Autodesk Inventor part; units mm, degrees
sketch "Skizze1" plane through (0, 0, 0) normal (0, 0, 1) x (1, 0, 0)
  line L0 (-9.4, 0) -> (56.4, 0)
  line L1 (0, -37.2) -> (0, 6.2)
  line L2 (0, 0) -> (47, 0)
  line L3 (47, 0) -> (47, -31)
  line L4 (47, -31) -> (0, -31)
  line L5 (0, -31) -> (0, 0)
  line L6 (5, -5) -> (42, -5)
  line L7 (42, -5) -> (42, -25)
  line L8 (42, -25) -> (39, -25)
  line L9 (39, -25) -> (39, -18)
  line L10 (39, -18) -> (8, -18)
  line L11 (8, -18) -> (8, -25)
  line L12 (8, -25) -> (5, -25)
  line L13 (5, -25) -> (5, -5)
  dimension "d0" = 47
  dimension "d1" = 31
  dimension "d2" = 5
  dimension "d3" = 5
  dimension "d4" = 5
  dimension "d5" = 6
  dimension "d6" = 6
  dimension "d7" = 3
  dimension "d8" = 3
  dimension "d9" = 13
extrude "Extrusion1" add sketch "Skizze1" along normal blind 50
fillet "Rundung1" radius 1 2 edges at (8, -18, 25) (39, -18, 25)
sketch "Skizze4" plane through (0, -31, 0) normal (-1, 0, 0) x (0, 0, 1)
  line L0 (50, 31) -> (50, 0)
  line L1 (0, 31) -> (50, 31)
  circle A0 centre (25, 17) radius 1.8
  dimension "d41" = 25
  dimension "d42" = 14
  dimension "d43" = 3.6
hole "Bohrung3" at (0, -14, 25) direction (1, 0, 0) diameter 6.15 end through all
sketch "Skizze5" plane through (0, 0, 0) normal (0, 1, 0) x (1, 0, 0)
  line L0 (0, 0) -> (47, 0)
  line L1 (0, 0) -> (10, 0)
  line L2 (10, 0) -> (10, -50)
  line L3 (10, -50) -> (0, -50)
  line L4 (0, -50) -> (0, 0)
  line L5 (47, 0) -> (47, -50)
  line L6 (47, 0) -> (37, 0)
  line L7 (37, 0) -> (37, -50)
  line L8 (37, -50) -> (47, -50)
  line L9 (47, -50) -> (47, 0)
  dimension "d51" = 10
  dimension "d52" = 50
  dimension "d53" = 10
  dimension "d54" = 50
extrude "Extrusion4" add sketch "Skizze5" along normal blind 10
sketch "Skizze6" plane through (47, -31, 50) normal (1, 0, 0) x (0, 0, -1)
  line L0 (0, 41) -> (50, 41)
  line L1 (50, 41) -> (50, 0)
  line L2 (0, 0) -> (0, 41)
  point P0 (50, 31)
  point P1 (12.5, 36)
  point P2 (25, 36)
  point P3 (37.5, 36)
  dimension "d57" = 5
  dimension "d58" = 5
  dimension "d59" = 5
  dimension "d60" = 12.5
  dimension "d61" = 12.5
  dimension "d62" = 12.5
hole "Bohrung4" at (47, 5, 37.5) at (47, 5, 25) at (47, 5, 12.5) direction (-1, 0, 0) diameter 6.15 end through all
properties part number "NASA Objektträgerhalter (Südkorea)"
Work out the finished part from the listing and answer in its coordinate system (mm). A direction names the side the tool comes from. Give positions to 0.01 mm unless a question says otherwise; leave off trailing zeros. Order: outer loops, then holes, each group sorted by start corner. A loop starts at its lowest first (then second) coordinate and runs counter-clockwise, first axis right, second up. Notation, with made-up numbers: (6.25, 43.5) - (24.25, 43.5) arc R15 cw to (24.25, 51.5) - close; hole circle Ø3 at (-11, -40). An arc over 180 degrees is marked (long way). Answer as CSV lines item,"result". Start each with the question number.
Q1. The part is cut by section C-C (z = 12.5). Write down the section's boundary in (x, y) (3 decimals), then the cut area to 3 significant figures.
Q2. Given pin 1 Ø8.5 at (x, z) = (24, 19) entering from +Y, flat-ended and moving along its own axis, determine where the tip first touches the part or whether it passes through.
Q3. The part is cut by section B-B (y = -8). Write down the section's boundary in (x, z).
Q4. The part is cut by section D-D (z = 4). Write down the section's boundary in (x, y), then the cut area to 3 significant figures.
Q5. The part is cut by section A-A (x = 41). Write down the section's boundary in (y, z) (3 decimals).
Q6. Find the intervals of material crossed by L1, parallel to Z at x = 6.5, y = 5 (3 decimals); L2, parallel to Y at x = 1.7, z = 25 (3 decimals); L3, parallel to X at y = -21, z = 7, in increasing order. Write a range as [from, to].
Q7. For faces 1 (the face through (7, -25, 25)), 2 (the face through (44.54, -14.14, 21.93)), 3 (the face through (37, 1.6, 24.7)), determine the directions among +Z, -Z, +X, -X, +Y, -Y from which every point of the face is accessible in a straight line to the end or side of a thin tool.
Q8. The mould has two halves that part along Y. Classify faces 4 (the face through (23, -19, 50)), 5 (the face through (24, -31, 25)), 6 (the face through (5, 10, 25)), 7 (the face through (24, -18, 25)): +Y half, -Y half, draft (parallel to the pull), parting line (faces both ways), or undercut.
Check result:
1,outline,"(0, -31) - (47, -31) - (47, 1.925) - (37, 1.925) - (37, 0) - (10, 0) - (10, 1.925) - (0, 1.925) - close; (0, 8.075) - (10, 8.075) - (10, 10) - (0, 10) - close; (37, 8.075) - (47, 8.075) - (47, 10) - (37, 10) - close; hole (5, -25) - (8, -25) - (8, -19) arc R1 cw to (9, -18) - (38, -18) arc R1 cw to (39, -19) - (39, -25) - (42, -25) - (42, -5) - (5, -5) - close"
1,area,"1,010 mm²"
2,pin 1,"stops at y = 0"
3,outline,"(0, 0) - (5, 0) - (5, 50) - (0, 50) - close; (42, 0) - (47, 0) - (47, 50) - (42, 50) - close"
4,outline,"(0, -31) - (47, -31) - (47, 10) - (37, 10) - (37, 0) - (10, 0) - (10, 10) - (0, 10) - close; hole (5, -25) - (8, -25) - (8, -19) arc R1 cw to (9, -18) - (38, -18) arc R1 cw to (39, -19) - (39, -25) - (42, -25) - (42, -5) - (5, -5) - close"
4,area,"1,130 mm²"
5,outline,"(-31, 0) - (-25, 0) - (-25, 50) - (-31, 50) - close; (-5, 0) - (10, 0) - (10, 50) - (-5, 50) - close; hole circle Ø6.15 at (5, 12.5); hole circle Ø6.15 at (5, 25); hole circle Ø6.15 at (5, 37.5)"
6,L1,"z = [0, 9.425], [15.575, 21.925], [28.075, 34.425], [40.575, 50]"
6,L2,"y = [-31, -17.075], [-10.925, 1.925], [8.075, 10]"
6,L3,"x = [0, 5], [8, 39], [42, 47]"
7,face 1,"+Z, -Z"
7,face 2,"+X, -X"
7,face 3,"+Z, -Z, +Y"
8,face 4,"draft"
8,face 5,"-Y half"
8,face 6,"+Y half"
8,face 7,"undercut"
